Model file for the job. Use its own axes, mm. A direction names the side the tool comes from. Give positions to 0.01 mm unless a question says otherwise; leave off trailing zeros. Loops run counter-clockwise (first coordinate to the right, second up) from the corner with the lowest first, then second, coordinate; pieces in that order, holes last. Notation, with made-up numbers: (74.5, -7) -> (105.5, -7) arc R10 ccw to (105.5, 2) -> close; hole circle Ø11 at (42, 76). An arc over 180 degrees is marked (long way). Use CSV: the item, a comma, the result in double quotes. Start each with the question number.
(1) Cut at A-A on z = 0. Write the cut outline in (x, y) (3 decimals).
(2) Flat gauge pins, fed straight in: pin 1 (1.5 mm diameter, centred on x = 7, y = 5.5, fed in from +Z); pin 2 (1.5 mm diameter, centred on x = 12.5, z = -6, fed in from -Y); pin 3 (1.5 mm diameter, centred on x = 5, y = -3.5, fed in from +Z). Where does each tip first touch, or does it go through?
(3) Pull direction Y, two halves, no side cores. Call faces 3 (the flat face through (8, 3.302, 0)), 4 (the flat face through (0, 5, 0)), 5 (the cylindrical face through (7.522, -7.555, -0.992)), 6 (the flat face through (8, -3.302, 0)): pulls with the +Y half, pulls with the -Y half, needs draft (parallel to the pull), parting line crosses it, or undercut.
(4) Cut at C-C on x = 12.75. Write the cut outline in (y, z).
(5) 3-axis set-ups, long thin cutter, end or side, ignore diameter. For faces 1 (the flat face through (15.24, 5, 0)), 2 (the flat face through (8, 0, -3.302)): which of +Z, -Z, +X, -X, +Y, -Y reach the whole face in a straight line?
(6) Drill centre lines: probe 1 along Y at (x, z) = (7.5, 0.25); probe 2 along Y at (x, z) = (12, -1.25); probe 3 along Z at (x, y) = (12, -1.5). Where is each one in solid material? Low to high.
from build123d import *

# Parameters (mm, degrees)
SKETCH1_R           = 7.62
SKETCH1_W           = 6.604
SKETCH1_H           = 6.604
BOSS_EXTRUDE1_DEPTH = 15.24
FILLET1_R           = 0.635


with BuildPart() as part:
    # Sketch1 → Boss-Extrude1 (new body)
    with BuildSketch(Plane(origin=(0, 0, 0), x_dir=(0, 0, -1), z_dir=(1, 0, 0))):
        with Locations(Location((0, 0, 0), (0, 0, 180))):
            Circle(SKETCH1_R)
        Rectangle(SKETCH1_W, SKETCH1_H, mode=Mode.SUBTRACT)
    extrude(amount=BOSS_EXTRUDE1_DEPTH)

    # Fillet1
    fillet1_edges = [part.edges().sort_by_distance(p)[0] for p in [
        (15.24, 0, 3.302),
        (15.24, -3.302, 0),
        (0, 0, -7.62),
        (15.24, 0, -7.62),
        (0, 0, -3.302),
        (0, 3.302, 0),
        (0, 0, 3.302),
        (0, -3.302, 0),
        (15.24, 0, -3.302),
        (15.24, 3.302, 0),
    ]]
    fillet(fillet1_edges, radius=FILLET1_R)


solid = part.part
Check result:
1,outline,"(0, -6.985) arc R0.635 ccw to (0.635, -7.62) -> (14.605, -7.62) arc R0.635 ccw to (15.24, -6.985) -> (15.24, -3.937) arc R0.635 ccw to (14.605, -3.302) -> (0.635, -3.302) arc R0.635 ccw to (0, -3.937) -> close; (0, 3.937) arc R0.635 ccw to (0.635, 3.302) -> (14.605, 3.302) arc R0.635 ccw to (15.24, 3.937) -> (15.24, 6.985) arc R0.635 ccw to (14.605, 7.62) -> (0.635, 7.62) arc R0.635 ccw to (0, 6.985) -> close"
2,pin 1,"z = 5.96"
2,pin 2,"y = -5.52"
2,pin 3,"z = 7.11"
3,face 3,"undercut"
3,face 4,"needs draft"
3,face 5,"parting line crosses it"
3,face 6,"undercut"
4,outline,"circle Ø15.24 at (0, 0); hole (-3.3, -3.3) -> (3.3, -3.3) -> (3.3, 3.3) -> (-3.3, 3.3) -> close"
5,face 1,"+Z, -Z, +X, +Y, -Y"
5,face 2,"+X, -X"
6,probe 1,"-7.62 to -3.3, 3.3 to 7.62"
6,probe 2,"-7.52 to -3.3, 3.3 to 7.52"
6,probe 3,"-7.47 to -3.3, 3.3 to 7.47"
